from build123d import *

# Parameters (mm, degrees)
SKETCH1_W           = 5
SKETCH1_H           = 5
BOSS_EXTRUDE2_DEPTH = 8
SKETCH1_4_W         = 90
SKETCH1_4_H         = 77.5
BOSS_EXTRUDE3_DEPTH = 3
SKETCH4_W           = 38
SKETCH4_H           = 43
CUT_EXTRUDE2_DEPTH  = 3


with BuildPart() as part:
    # Sketch1 → Boss-Extrude2 (new body)
    with BuildSketch(Plane.XY):
        with Locations((7.5, 7.5)):
            Rectangle(SKETCH1_W, SKETCH1_H)
        with Locations((7.5, 12.5)):
            Rectangle(SKETCH1_W, SKETCH1_H)
        with Locations((12.5, 7.5)):
            Rectangle(SKETCH1_W, SKETCH1_H)
        with Locations((7.5, 70.5)):
            Rectangle(SKETCH1_W, SKETCH1_H)
        Polygon((10, 63), (10, 68), (5, 68), (5, 65.122658067), (5, 63), align=None)
        with Locations((12.5, 70.5)):
            Rectangle(SKETCH1_W, SKETCH1_H)
        with Locations((60.5, 70.5)):
            Rectangle(SKETCH1_W, SKETCH1_H)
        with Locations((65.5, 70.5)):
            Rectangle(SKETCH1_W, SKETCH1_H)
        with Locations((65.5, 65.5)):
            Rectangle(SKETCH1_W, SKETCH1_H)
        with Locations((65.5, 12.5)):
            Rectangle(SKETCH1_W, SKETCH1_H)
        with Locations((65.5, 7.5)):
            Rectangle(SKETCH1_W, SKETCH1_H)
        with Locations((60.5, 7.5)):
            Rectangle(SKETCH1_W, SKETCH1_H)
    extrude(amount=BOSS_EXTRUDE2_DEPTH)

    # Sketch1_4 → Boss-Extrude3 (add)
    with BuildSketch(Plane.XY):
        with Locations((45, 38.75)):
            Rectangle(SKETCH1_4_W, SKETCH1_4_H)
        Polygon((15, 5), (5, 5), (5, 15), (10, 15), (10, 10), (15, 10), align=None, mode=Mode.SUBTRACT)
        Polygon((58, 5), (58, 10), (63, 10), (63, 15), (68, 15), (68, 5), align=None, mode=Mode.SUBTRACT)
        Polygon((5, 63), (5, 73), (15, 73), (15, 68), (10, 68), (10, 63), align=None, mode=Mode.SUBTRACT)
        Polygon((63, 68), (58, 68), (58, 73), (68, 73), (68, 63), (63, 63), align=None, mode=Mode.SUBTRACT)
    extrude(amount=BOSS_EXTRUDE3_DEPTH)

    # Sketch4 → Cut-Extrude2 (cut)
    with BuildSketch(Plane.XY.offset(3)):
        with Locations((36.5, 39)):
            Rectangle(SKETCH4_W, SKETCH4_H)
    extrude(amount=-CUT_EXTRUDE2_DEPTH, mode=Mode.SUBTRACT)


solid = part.part
Geometry check sheet. Reference: the model listing, model coordinates, mm. A direction names the side the tool comes from. Round coordinates to 2 decimals unless told otherwise and drop trailing zeros. Order: outer loops, then holes, each group sorted by start corner. A loop starts at its lowest first (then second) coordinate and runs counter-clockwise, first axis right, second up. Notation, with made-up numbers: M -5,57 L 27,57 A11 ccw 27,76 Z; hole C 76,9 d7. An arc over 180 degrees is marked long. Answer in a Markdown table with one row per item.
(1) Go/stop test with flat-tipped pins: P1, Ø4, axis at y = 7, z = 6, coming from the +X side; P2, Ø6, axis at x = 75, y = 30, coming from the +Z side; P3, Ø1.5, axis at x = 13.5, z = 4.5, coming from the -Y side. Record where each tip stops, or that it passes through.
Responses:
| item | result |
|---|---|
| P1 | stops at x = 68 |
| P2 | stops at z = 3 |
| P3 | stops at y = 5 |
(2) Scan lines: probe 1 along Y at (x, z) = (53.5, 2.5); probe 2 along X at (y, z) = (32, 2.5); probe 3 along Z at (x, y) = (76, 41). Record each from-to range of solid material in increasing order. Write a range as from..to.
Responses:
| item | result |
|---|---|
| probe 1 | y = 0..17.5, 60.5..77.5 |
| probe 2 | x = 0..17.5, 55.5..90 |
| probe 3 | z = 0..3 |
(3) Tool access check on faces 5 (the face through (5, 68, 5)), 6 (the face through (12, 10, 5)), 7 (the face through (7, 63, 5)), 8 (the face through (15, 7, 5)), 9 (the face through (10, 73, 5)). Record the directions out of +Z, -Z, +X, -X, +Y, -Y that give a thin tool (end or side, any length) a straight path to the whole face; none if there is none.
Responses:
| item | result |
|---|---|
| face 5 | +Z, -X, +Y, -Y |
| face 6 | +Z |
| face 7 | +Z, +X, -X |
| face 8 | +Z, +Y, -Y |
| face 9 | +Z, +X, -X, +Y |
(4) Sectioned sample at B-B, the plane x = 34.5. Record the cut outline in (y, z).
Responses:
| item | result |
|---|---|
| outline | M 0,0 L 17.5,0 L 17.5,3 L 0,3 Z; M 60.5,0 L 77.5,0 L 77.5,3 L 60.5,3 Z |
(5) Draft check along X on faces 1 (the face through (68, 68, 5)), 2 (the face through (9, 69, 8)), 3 (the face through (55.5, 39, 2)), 4 (the face through (5, 10, 5)). Enter one of: released by +X, released by -X, zero draft, split by the parting line, or undercut.
Responses:
| item | result |
|---|---|
| face 1 | released by +X |
| face 2 | zero draft |
| face 3 | undercut |
| face 4 | released by -X |
(6) Sectioned sample at C-C, the plane z = 7. Record the cut outline in (x, y).
Responses:
| item | result |
|---|---|
| outline | M 5,5 L 15,5 L 15,10 L 10,10 L 10,15 L 5,15 Z; M 5,63 L 10,63 L 10,68 L 15,68 L 15,73 L 5,73 Z; M 58,5 L 68,5 L 68,15 L 63,15 L 63,10 L 58,10 Z; M 58,68 L 63,68 L 63,63 L 68,63 L 68,73 L 58,73 Z |
(7) Sectioned sample at D-D, the plane z = 1. Record the cut outline in (x, y), and give its area (3 significant figures).
Responses:
| item | result |
|---|---|
| outline | M 0,0 L 90,0 L 90,77.5 L 0,77.5 Z; hole M 17.5,17.5 L 55.5,17.5 L 55.5,60.5 L 17.5,60.5 Z |
| area | 5,340 mm² |
(8) Sectioned sample at A-A, the plane y = 38. Record the cut outline in (x, z), and give its area (3 significant figures).
Responses:
| item | result |
|---|---|
| outline | M 0,0 L 17.5,0 L 17.5,3 L 0,3 Z; M 55.5,0 L 90,0 L 90,3 L 55.5,3 Z |
| area | 156 mm² |
